Verification items for the finished model (mm, model axes). Face numbers are marked on the shaded views. A direction names the side the tool comes from. Round coordinates to 2 decimals unless told otherwise and drop trailing zeros. Order: outer loops, then holes, each group sorted by start corner. A loop starts at its lowest first (then second) coordinate and runs counter-clockwise, first axis right, second up. Notation, with made-up numbers: (-5.75, -5.75) -> (23.25, -5.75) arc R18 ccw to (23.25, 7.25) -> close; hole circle Ø9 at (55.25, 32). An arc over 180 degrees is marked (long way). Put each result on its own line as item: value.
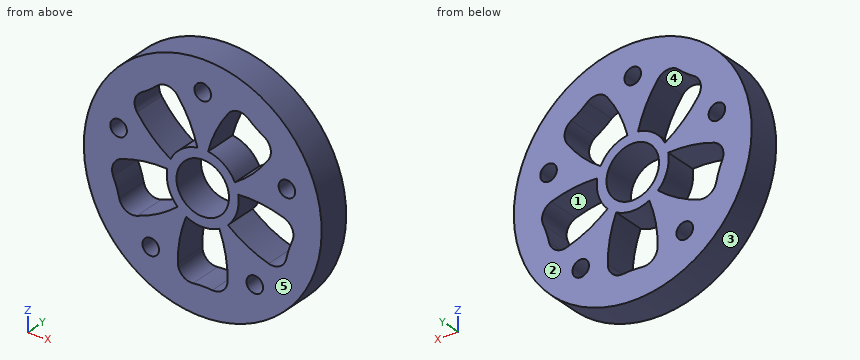
```python
from build123d import *

# Parameters (mm, degrees)
SKETCH_1_R          = 43
SKETCH_1_R_2        = 3
EXTRUDE_1_DEPTH     = 12
SKETCH_2_R          = 9.5
CUT_EXTRUDE_1_DEPTH = 62.983868869


with BuildPart() as part:
    # 草图1 → 凸台-拉伸1 (new body)
    with BuildSketch(Plane(origin=(0, 0, 0), x_dir=(1, 0, 0), z_dir=(0, 1, 0))):
        with Locations(Location((0, 0, 0), (0, 0, 270))):
            Circle(SKETCH_1_R)
        with Locations(Location((0, -32, 0), (0, 0, 270))):
            Circle(SKETCH_1_R_2, mode=Mode.SUBTRACT)
        with Locations(Location((-30.433808521, -9.88854382, 0), (0, 0, 270))):
            Circle(SKETCH_1_R_2, mode=Mode.SUBTRACT)
        with Locations(Location((-18.809128073, 25.88854382, 0), (0, 0, 270))):
            Circle(SKETCH_1_R_2, mode=Mode.SUBTRACT)
        with Locations(Location((18.809128073, 25.88854382, 0), (0, 0, 270))):
            Circle(SKETCH_1_R_2, mode=Mode.SUBTRACT)
        with Locations(Location((30.433808521, -9.88854382, 0), (0, 0, 270))):
            Circle(SKETCH_1_R_2, mode=Mode.SUBTRACT)
    extrude(amount=EXTRUDE_1_DEPTH)

    # 草图2 → 切除-拉伸1 (cut, through all)
    with BuildSketch(Plane(origin=(0, 12, 0), x_dir=(1, 0, 0), z_dir=(0, 1, 0))):
        with Locations(Location((0, 0, 0), (0, 0, 270))):
            Circle(SKETCH_2_R)
        with BuildLine():
            ThreePointArc((6, 11.532562595), (0, 13), (-6, 11.532562595))
            ThreePointArc((-6, 11.532562595), (-8.308699922, 19.618928286), (-8.999382438, 28))
            ThreePointArc((-8.999382438, 28), (-7.324858249, 31.655760291), (-3.5, 32.896354479))
            ThreePointArc((-3.5, 32.896354479), (0, 32.720914778), (3.5, 32.896354479))
            ThreePointArc((3.5, 32.896354479), (7.324858249, 31.655760291), (8.999382438, 28))
            ThreePointArc((8.999382438, 28), (8.308699922, 19.618928286), (6, 11.532562595))
        make_face()
        with BuildLine():
            ThreePointArc((12.822220771, -2.142581267), (12.363734712, 4.017220927), (9.114016839, 9.270096928))
            ThreePointArc((9.114016839, 9.270096928), (16.091180112, 13.964625454), (23.848620344, 17.211397152))
            ThreePointArc((23.848620344, 17.211397152), (27.842911423, 16.748522069), (30.204732809, 13.494230394))
            ThreePointArc((30.204732809, 13.494230394), (31.119439219, 10.111318738), (32.36785177, 6.83683478))
            ThreePointArc((32.36785177, 6.83683478), (32.369922784, 2.815813731), (29.410544568, 0.093554533))
            ThreePointArc((29.410544568, 0.093554533), (21.226239066, -1.839460951), (12.822220771, -2.142581267))
        make_face()
        with BuildLine():
            ThreePointArc((1.924568248, -12.856750642), (7.64120828, -10.517220927), (11.632772181, -5.803327614))
            ThreePointArc((11.632772181, -5.803327614), (18.25359615, -10.988315115), (23.738640395, -17.362771566))
            ThreePointArc((23.738640395, -17.362771566), (24.532723854, -21.304604391), (22.167551497, -24.556461444))
            ThreePointArc((22.167551497, -24.556461444), (19.232871148, -26.471776127), (16.504432537, -28.67095821))
            ThreePointArc((16.504432537, -28.67095821), (12.680854244, -29.915491699), (9.177333733, -27.942180119))
            ThreePointArc((9.177333733, -27.942180119), (4.809837274, -20.755777674), (1.924568248, -12.856750642))
        make_face()
        with BuildLine():
            ThreePointArc((-11.632772181, -5.803327614), (-7.64120828, -10.517220927), (-1.924568248, -12.856750642))
            ThreePointArc((-1.924568248, -12.856750642), (-4.809837274, -20.755777674), (-9.177333733, -27.942180119))
            ThreePointArc((-9.177333733, -27.942180119), (-12.680854244, -29.915491699), (-16.504432537, -28.67095821))
            ThreePointArc((-16.504432537, -28.67095821), (-19.232871148, -26.471776127), (-22.167551497, -24.556461444))
            ThreePointArc((-22.167551497, -24.556461444), (-24.532723854, -21.304604391), (-23.738640395, -17.362771566))
            ThreePointArc((-23.738640395, -17.362771566), (-18.25359615, -10.988315115), (-11.632772181, -5.803327614))
        make_face()
        with BuildLine():
            ThreePointArc((-9.114016839, 9.270096928), (-12.363734712, 4.017220927), (-12.822220771, -2.142581267))
            ThreePointArc((-12.822220771, -2.142581267), (-21.226239066, -1.839460951), (-29.410544568, 0.093554533))
            ThreePointArc((-29.410544568, 0.093554533), (-32.369922784, 2.815813731), (-32.36785177, 6.83683478))
            ThreePointArc((-32.36785177, 6.83683478), (-31.119439219, 10.111318738), (-30.204732809, 13.494230394))
            ThreePointArc((-30.204732809, 13.494230394), (-27.842911423, 16.748522069), (-23.848620344, 17.211397152))
            ThreePointArc((-23.848620344, 17.211397152), (-16.091180112, 13.964625454), (-9.114016839, 9.270096928))
        make_face()
    extrude(amount=-CUT_EXTRUDE_1_DEPTH, mode=Mode.SUBTRACT)


solid = part.part
```
Item 1: Sectioned sample at B-B, the plane z = -24. Record the boundary of the cut face in (x, y).
Geometry check:
outline: (-35.68, 0) -> (-21.14, 0) -> (-21.14, 12) -> (-35.68, 12) -> close; (-16.48, 0) -> (-8.88, 0) -> (-8.88, 12) -> (-16.48, 12) -> close; (8.88, 0) -> (16.48, 0) -> (16.48, 12) -> (8.88, 12) -> close; (21.14, 0) -> (35.68, 0) -> (35.68, 12) -> (21.14, 12) -> close
Item 2: Release check for a two-part mould opening along X. For the marked faces 3, 4 and 5 record: pulls with the +X half, pulls with the -X half, needs draft (parallel to the pull), parting line crosses it, or undercut.
Geometry check:
face 3: parting line crosses it
face 4: undercut
face 5: needs draft
Item 3: Material ranges on line 1 along Z through (x, y) = (-23, 10.5); line 2 along X through (y, z) = (6.75, 14.5); line 3 along Z through (x, y) = (-17, 5.5), recorded low to high.
Geometry check:
line 1: -36.33 to -16.94, 1.56 to 16.34, 23.95 to 36.33
line 2: -40.48 to -21.54, -2.38 to 2.38, 21.54 to 40.48
line 3: -39.5 to -28.28, -23.5 to -14.44, 2.2 to 9.84, 28.24 to 39.5
Item 4: Sectioned sample at D-D, the plane y = 6.25. Give the number of separate pieces and of enclosed holes in the cut face, then the cut area to 3 significant figures.
Geometry check:
separate pieces: 1
enclosed holes: 11
area: 3,730 mm2
Item 5: Depth check by flat-ended pin: pin 1 Ø17 at (x, z) = (0, 0) entering from +Y; pin 2 Ø2 at (x, z) = (32.5, 10) entering from +Y; pin 3 Ø3 at (y, z) = (1.5, 7.5) entering from -X; pin 4 Ø1.5 at (y, z) = (10.5, -26) entering from +X. Enter the tip coordinate at first touch or a pass-through.
Geometry check:
pin 1: through
pin 2: y = 12
pin 3: x = -42.58
pin 4: x = 34.81
Item 6: Sectioned sample at C-C, the plane z = 32. Record the boundary of the cut face in (x, y).
Geometry check:
outline: (-28.72, 0) -> (-3, 0) -> (-3, 12) -> (-28.72, 12) -> close; (3, 0) -> (28.72, 0) -> (28.72, 12) -> (3, 12) -> close
Item 7: Sectioned sample at A-A, the plane x = 0. Record the boundary of the cut face in (y, z).
Geometry check:
outline: (0, -43) -> (12, -43) -> (12, -32.72) -> (0, -32.72) -> close; (0, -13) -> (12, -13) -> (12, -9.5) -> (0, -9.5) -> close; (0, 9.5) -> (12, 9.5) -> (12, 29) -> (0, 29) -> close; (0, 35) -> (12, 35) -> (12, 43) -> (0, 43) -> close
Item 8: Tool access check on the marked faces 1 and 2. Record the directions out of +Z, -Z, +X, -X, +Y, -Y that give a thin tool (end or side, any length) a straight path to the whole face; none if there is none.
Geometry check:
face 1: +Y, -Y
face 2: +Z, -Z, +X, -X, +Y
